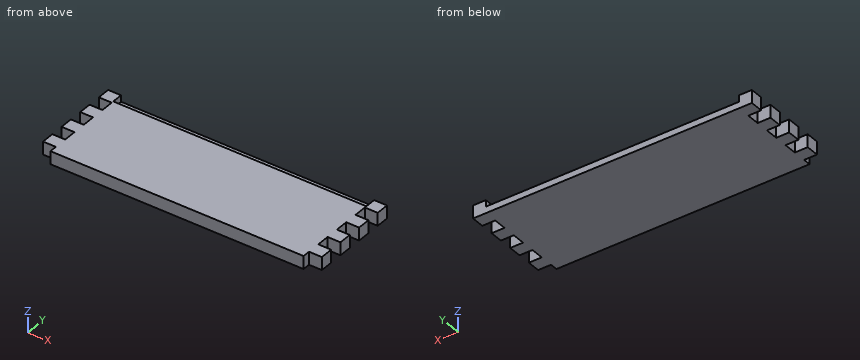
Autodesk Inventor part; units mm, degrees
ref_plane "YZ Plane" through (0, 0, 0) normal (1, 0, 0) x (0, 1, 0)
ref_plane "XZ Plane" through (0, 0, 0) normal (0, 1, 0) x (-1, 0, 0)
ref_plane "XY Plane" through (0, 0, 0) normal (0, 0, 1) x (1, 0, 0)
sketch "Sketch1" plane through (0, 0, 0) normal (0, 0, 1) x (1, 0, 0)
  line L0 (0, 244.475) -> (19.05, 244.475)
  line L1 (19.05, 244.475) -> (19.05, 225.425)
  line L2 (19.05, 225.425) -> (0, 225.425)
  line L3 (0, 225.425) -> (0, 244.475)
  line L4 (19.05, 168.275) -> (0, 168.275)
  line L5 (0, 168.275) -> (0, 149.225)
  line L6 (0, 149.225) -> (19.05, 149.225)
  line L7 (19.05, 149.225) -> (19.05, 168.275)
  line L8 (0, 130.175) -> (19.05, 130.175)
  line L9 (19.05, 130.175) -> (19.05, 111.125)
  line L10 (19.05, 111.125) -> (0, 111.125)
  line L11 (0, 111.125) -> (0, 130.175)
  line L12 (0, 206.375) -> (19.05, 206.375)
  line L13 (19.05, 206.375) -> (19.05, 187.325)
  line L14 (19.05, 187.325) -> (0, 187.325)
  line L15 (0, 187.325) -> (0, 206.375)
  line L16 (0, 92.075) -> (19.05, 92.075)
  line L17 (19.05, 92.075) -> (19.05, 73.025)
  line L18 (19.05, 73.025) -> (0, 73.025)
  line L19 (0, 73.025) -> (0, 92.075)
  line L20 (0, 53.975) -> (19.05, 53.975)
  line L21 (19.05, 53.975) -> (19.05, 34.925)
  line L22 (19.05, 34.925) -> (0, 34.925)
  line L23 (0, 34.925) -> (0, 53.975)
  line L24 (0, 15.875) -> (19.05, 15.875)
  line L25 (19.05, 15.875) -> (19.05, -3.175)
  line L26 (19.05, -3.175) -> (0, -3.175)
  line L27 (0, -3.175) -> (0, 15.875)
  line L28 (0, 244.475) -> (206.375, 244.475)
  line L29 (206.375, 244.475) -> (206.375, 76.2)
  line L30 (206.375, 76.2) -> (0, 76.2)
  line L31 (19.05, 244.475) -> (19.05, 76.2)
  line L32 (206.375, 244.475) -> (19.05, 244.475)
  line L33 (19.05, 244.475) -> (19.05, 76.2)
  line L34 (19.05, 76.2) -> (206.375, 76.2)
  line L35 (206.375, 76.2) -> (206.375, 244.475)
  line L36 (0, 92.075) -> (19.05, 92.075)
  line L37 (19.05, 92.075) -> (19.05, 76.2)
  line L38 (19.05, 76.2) -> (0, 76.2)
  line L39 (0, 76.2) -> (0, 92.075)
  dimension "d0" = 19.05
  dimension "d1" = 19.05
  dimension "d3" = 19.05
  dimension "d4" = 19.05
  dimension "d5" = 19.05
  dimension "d6" = 19.05
  dimension "d7" = 19.05
  dimension "d8" = 19.05
  dimension "d9" = 19.05
  dimension "d10" = 19.05
  dimension "d11" = 19.05
  dimension "d12" = 19.05
  dimension "d13" = 19.05
  dimension "d14" = 19.05
  dimension "d15" = 19.05
  dimension "d16" = 19.05
  dimension "d17" = 19.05
  dimension "d18" = 19.05
  dimension "d19" = 19.05
  dimension "d21" = 206.375
  dimension "d22" = 168.275
  dimension "d23" = 206.375
extrude "Extrusion3" add sketch "Sketch1" along normal blind 19.05 contours L0 L1 L2 L3 | L28 L29 L30 L17 L31 L9 L7 L13 L1 | L13 L14 L15 L12 | L30 L19 L16 L17 | L7 L6 L5 L4 | L10 L11 L8 L9
mirror "Mirror2" about plane through (206.375, 76.2, 0) normal (1, 0, 0) of "Extrusion3"
sketch "Sketch3" plane through (0, 0, 19.05) normal (0, 0, 1) x (1, 0, 0)
  line L0 (0, 244.475) -> (412.75, 244.475)
  line L1 (19.05, 244.475) -> (393.7, 244.475)
  line L2 (393.7, 244.475) -> (393.7, 228.6)
  line L3 (393.7, 228.6) -> (19.05, 228.6)
  line L4 (19.05, 228.6) -> (19.05, 244.475)
  point P0 (0, 0)
  dimension "d33" = 15.875
extrude "Extrusion4" cut sketch "Sketch3" against normal blind 9.525
sketch "Sketch4" plane through (0, 0, 19.05) normal (0, 0, 1) x (1, 0, 0)
  line L0 (0, 244.475) -> (19.05, 244.475)
  line L1 (19.05, 111.125) -> (19.05, 92.075)
  line L2 (19.05, 92.075) -> (0, 92.075)
  line L3 (0, 92.075) -> (0, 76.2)
  line L4 (0, 76.2) -> (412.75, 76.2)
  line L5 (412.75, 92.075) -> (412.75, 76.2)
  line L6 (393.7, 92.075) -> (412.75, 92.075)
  line L7 (393.7, 111.125) -> (393.7, 92.075)
  line L8 (19.05, 100.0125) -> (393.7, 100.0125)
  point P0 (0, 0)
  dimension "d36" = 144.4625
extrude "Extrusion5" cut sketch "Sketch4" against normal through all
properties part number "deep_end" material "Wood (Birch)"
Geometry check sheet. Reference: the model listing, model coordinates, mm. Round coordinates to 2 decimals unless told otherwise and drop trailing zeros. Order: outer loops, then holes, each group sorted by start corner. A loop starts at its lowest first (then second) coordinate and runs counter-clockwise, first axis right, second up. Notation, with made-up numbers: (3, 73.25) -> (45, 73.25) arc R18 ccw to (45, 89.25) -> close; hole circle Ø8 at (-34.75, 5). An arc over 180 degrees is marked (long way). Return JSON: item names as keys, results as strings. Group by question number.
Q1. Material ranges on probe 1 along X at (y, z) = (234.5, 12.75); probe 2 along X at (y, z) = (109, 4); probe 3 along Y at (x, z) = (132.5, 13), recorded low to high. Write a range as from..to.
Q2. Gauge pin test, flat ends, axial feed: pin 1 (17.5 mm diameter, centred on x = 113, y = 240, fed in from +Z) (3 decimals); pin 2 (5.5 mm diameter, centred on y = 214.5, z = 5, fed in from -X); pin 3 (5.5 mm diameter, centred on x = 8.5, z = 12.5, fed in from -Y) (3 decimals). Record the tip position at first contact, or that the pin passes through.
Q3. Section check C-C, the plane y = 213. Record the boundary of the cut face in (x, z).
Numbers:
{
 "1": {"probe 1": "0..19.05, 393.7..412.75", "probe 2": "19.05..393.7", "probe 3": "100.01..228.6"},
 "2": {"pin 1": "z = 9.525", "pin 2": "x = 19.05", "pin 3": "y = 111.125"},
 "3": {"outline": "(19.05, 0) -> (393.7, 0) -> (393.7, 19.05) -> (19.05, 19.05) -> close"}
}
